Could you check a few things on this model? Use its own coordinates, in mm. Face numbers are marked on the shaded views. A direction names the side the tool comes from. Give positions to 0.01 mm unless a question says otherwise; leave off trailing zeros. Order: outer loops, then holes, each group sorted by start corner. A loop starts at its lowest first (then second) coordinate and runs counter-clockwise, first axis right, second up. Notation, with made-up numbers: M 18,-7.75 L 52,-7.75 A25 ccw 52,26.25 Z; hole C 4,41.25 d6. An arc over 180 degrees is marked long. Use a Markdown table: item, result. Add a question column.
Item 1: Suppose I cut it at B-B on y = -9. Write out the boundary of the cut face in (x, z).
Item 2: Suppose I cut it at D-D on y = -22. Write out the boundary of the cut face in (x, z).
Item 3: For the marked faces 1, 2, 3 and 4, which set-ups out of +Z, -Z, +X, -X, +Y, -Y let a thin tool reach every point of the face, with its end or its side?
Item 4: If I drill on L1, parallel to Z at x = -123, y = -19; L2, parallel to Z at x = -120.5, y = -31; L3, parallel to Z at x = -142, y = -21.5, over which ranges is the centre line in solid material (lowest first)? Write a range as from..to.
Item 5: If we mould it in two halves opening along Z, with no side actions, what happens to the marked faces 5, 6 and 7? For each: released by +Z, released by -Z, zero draft, split by the parting line, or undercut.
Item 6: Suppose I cut it at A-A on z = -30.1. Write out the boundary of the cut face in (x, y), plus the area to 4 significant figures.
Item 7: I'm going to push flat-ended pins straight in: pin 1 Ø12 at (x, z) = (-129, -5) entering from +Y; pin 2 Ø1.3 at (x, y) = (-107, -17.5) entering from -Z; pin 3 Ø3 at (x, y) = (-147, -7.5) entering from +Z; pin 4 Ø5.5 at (x, z) = (-117.96, 1) entering from -Y. Where does each tip first touch, or does it pass through?
Item 8: Suppose I cut it at C-C on x = -129. Write out the boundary of the cut face in (y, z).
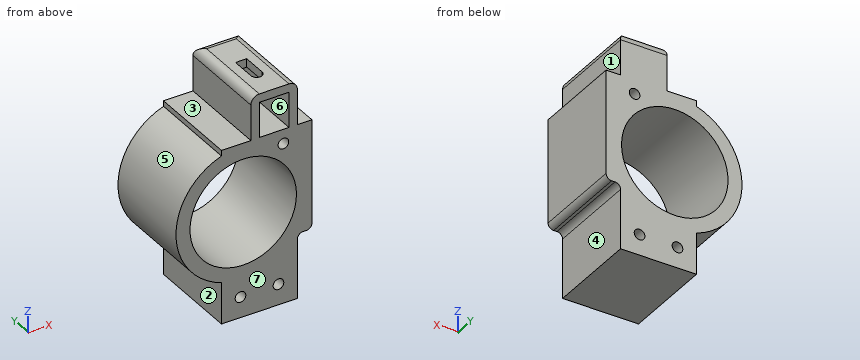
from build123d import *

# Parameters (mm, degrees)
F0_R      = 1.9
F0_R_2    = 19
F1_DEPTH  = 33
F2_W      = 10.6
F2_H      = 12.6
F3_DEPTH  = 6.7
F4_R      = 3
F5_R      = 2
F7_DEPTH  = 8.5
F8_R      = 1.99999
F9_R      = 2.15
F9_R_2    = 1
F10_DEPTH = 3
F11_DEPTH = 3.5


# Not quite as in the source:
# - a fillet or chamfer is up to 0.001 mm smaller than in the source, because OpenCascade refuses the exact size


with BuildPart() as f1:
    # F0 (on Front) → F1 (new body)
    with BuildSketch(Plane.XZ):
        with BuildLine():
            Line((-109.659200659, 0), (-109.659200659, 10.3))
            Line((-109.659200659, 10.3), (-126.259200659, 10.3))
            Line((-126.259200659, 10.3), (-126.259200659, 0))
            Line((-126.259200659, 0), (-126.259200659, -5))
            Line((-126.259200659, -5), (-126.259200659, -5.4))
            Line((-126.259200659, -5.4), (-136.75, -5.4))
            Line((-136.75, -5.4), (-136.75, -7.385742363))
            ThreePointArc((-136.75, -7.385742363), (-153, -30.1), (-136.75, -52.814257637))
            Line((-136.75, -52.814257637), (-136.75, -67.6))
            Line((-136.75, -67.6), (-132.812420773, -67.6))
            Line((-132.812420773, -67.6), (-109.659200659, -67.6))
            Line((-109.659200659, -67.6), (-109.659200659, -44.3103300754))
            Line((-109.659200659, -44.3103300754), (-105, -44.3103300754))
            Line((-105, -44.3103300754), (-104.5, -44.3103300754))
            Line((-104.5, -44.3103300754), (-104.5, -5.3))
            Line((-104.5, -5.3), (-105, -5.3))
            Line((-105, -5.3), (-109.659200659, -5.3))
            Line((-109.659200659, -5.3), (-109.659200659, 0))
        make_face()
        with Locations((-129.9773001648, -60.2071288185)):
            Circle(F0_R, mode=Mode.SUBTRACT)
        with Locations((-129, -30.1)):
            Circle(F0_R_2, mode=Mode.SUBTRACT)
        with Locations((-116.4319004943, -60.2071288185)):
            Circle(F0_R, mode=Mode.SUBTRACT)
        with Locations((-114.659200659, -10.3896699246)):
            Circle(F0_R, mode=Mode.SUBTRACT)
        Polygon((-112.659200659, -5.3), (-117.959200659, -5.3), (-123.259200659, -5.3), (-123.259200659, 7.3), (-112.659200659, 7.3), align=None, mode=Mode.SUBTRACT)
    extrude(amount=F1_DEPTH)

    # F2 (on face) → F3 (join)
    with BuildSketch(Plane(origin=(0, 0, 0), x_dir=(-1, 0, 0), z_dir=(0, 1, 0))):
        with Locations((117.959200659, 1)):
            Rectangle(F2_W, F2_H)
    extrude(amount=-F3_DEPTH)

    # F4
    f4_edges = [f1.edges().sort_by_distance(p)[0] for p in [
        (-109.659201, -16.5, 10.3),
        (-126.259201, -16.5, 10.3),
        (-117.959201, 0, 10.3),
    ]]
    fillet(f4_edges, radius=F4_R)

    # F5
    f5_edges = [f1.edges().sort_by_distance(p)[0] for p in [
        (-104.5, -16.5, -44.31033),
        (-109.659201, -16.5, -44.31033),
    ]]
    fillet(f5_edges, radius=F5_R)

    # F6 (on face) → F7 (cut)
    with BuildSketch(Plane.XY.offset(10.3)):
        Polygon((-119.959200659, -25), (-117.959200659, -25), (-115.959200659, -25), (-115.959200659, -14.2), (-119.959200659, -14.2), align=None)
    extrude(amount=-F7_DEPTH, mode=Mode.SUBTRACT)

    # F8 (radius 2 in the source; OpenCascade refuses exactly that, so slightly less here)
    f8_edges = [f1.edges().sort_by_distance(p)[0] for p in [
        (-119.959201, -25, 8.8),
        (-115.959201, -25, 8.8),
    ]]
    fillet(f8_edges, radius=F8_R)

    # F9 (on face) → F10 (cut)
    with BuildSketch(Plane.XZ.offset(6.7)):
        with Locations((-117.959200659, 1)):
            Circle(F9_R)
        with Locations((-117.959200659, 1)):
            Circle(F9_R_2, mode=Mode.SUBTRACT)
    extrude(amount=-F10_DEPTH, mode=Mode.SUBTRACT)

    # F11 (add): a face of the model
    f11_faces = [f1.faces().sort_by_distance(p)[0] for p in [
        (-117.959200659, -6.7, 1),
    ]]
    extrude(f11_faces, amount=F11_DEPTH)


solid = f1.part
Findings below:
| question | item | result |
|---|---|---|
| 1 | outline | M -136.75,-67.6 L -109.66,-67.6 L -109.66,-46.31 A2 cw -107.66,-44.31 L -106.5,-44.31 A2 ccw -104.5,-42.31 L -104.5,-5.3 L -109.66,-5.3 L -109.66,7.3 A3 ccw -112.66,10.3 L -123.26,10.3 A3 ccw -126.26,7.3 L -126.26,-5.4 L -136.75,-5.4 L -136.75,-7.39 A24 ccw -136.75,-52.81 Z; C -117.96,1 d2; hole C -129,-30.1 d38; hole C -129.98,-60.21 d3.8; hole M -123.26,-5.3 L -112.66,-5.3 L -112.66,7.3 L -123.26,7.3 Z; hole C -116.43,-60.21 d3.8; hole C -114.66,-10.39 d3.8 |
| 2 | outline | M -136.75,-67.6 L -109.66,-67.6 L -109.66,-46.31 A2 cw -107.66,-44.31 L -106.5,-44.31 A2 ccw -104.5,-42.31 L -104.5,-5.3 L -109.66,-5.3 L -109.66,7.3 A3 ccw -112.66,10.3 L -115.96,10.3 L -115.96,7.3 L -112.66,7.3 L -112.66,-5.3 L -123.26,-5.3 L -123.26,7.3 L -119.96,7.3 L -119.96,10.3 L -123.26,10.3 A3 ccw -126.26,7.3 L -126.26,-5.4 L -136.75,-5.4 L -136.75,-7.39 A24 ccw -136.75,-52.81 Z; hole C -129,-30.1 d38; hole C -129.98,-60.21 d3.8; hole C -116.43,-60.21 d3.8; hole C -114.66,-10.39 d3.8 |
| 3 | face 1 | +Z, +X, +Y, -Y |
| 3 | face 2 | -Z, -X, +Y, -Y |
| 3 | face 3 | +Z, -X, +Y, -Y |
| 3 | face 4 | -Z, +X, +Y, -Y |
| 4 | L1 | z = -67.6..-48.13, -12.07..-5.3, 7.3..10.3 |
| 4 | L2 | z = -67.6..-47.09, -13.11..-5.3, 7.3..10.3 |
| 4 | L3 | z = -50.27..-43.96, -16.24..-9.93 |
| 5 | face 5 | split by the parting line |
| 5 | face 6 | undercut |
| 5 | face 7 | zero draft |
| 6 | outline | M -153,-33 L -148,-33 L -148,0 L -153,0 Z; M -110,-33 L -104.5,-33 L -104.5,0 L -110,0 Z |
| 6 | area | 346.5 mm^2 |
| 7 | pin 1 | stops at y = 0 |
| 7 | pin 2 | stops at z = -44.31 |
| 7 | pin 3 | stops at z = -12.67 |
| 7 | pin 4 | stops at y = -10.2 |
| 8 | outline | M -33,-67.6 L 0,-67.6 L 0,-61.84 L -33,-61.84 Z; M -33,-58.58 L 0,-58.58 L 0,-49.1 L -33,-49.1 Z; M -33,-11.1 L 0,-11.1 L 0,-5.4 L -33,-5.4 Z |
